```python
from build123d import *

# Parameters (mm, degrees)
F0_R      = 16
F0_R_2    = 15
F1_DEPTH  = 5
F2_R      = 16
F3_DEPTH  = 2
F4_R      = 3
F5_R      = 16
F6_DEPTH  = 1
F7_R      = 3
F8_R      = 5
F9_DEPTH  = 7
F10_R     = 6.15
F10_R_2   = 5.75
F11_DEPTH = 5


with BuildPart() as f1:
    # F0 (on Top) → F1 (new body)
    with BuildSketch(Plane.XY):
        Circle(F0_R)
        Circle(F0_R_2, mode=Mode.SUBTRACT)
    extrude(amount=F1_DEPTH)

    # F2 (on face) → F3 (join)
    with BuildSketch(Plane.XY.offset(5)):
        Circle(F2_R)
    extrude(amount=F3_DEPTH)

    # F4
    f4_edges = [f1.edges().sort_by_distance(p)[0] for p in [
        (-16, 0, 7),
    ]]
    fillet(f4_edges, radius=F4_R)

    # F5 (on face) → F6 (join)
    with BuildSketch(Plane(origin=(0, 0, 0), x_dir=(1, 0, 0), z_dir=(0, 0, -1))):
        Circle(F5_R)
    extrude(amount=F6_DEPTH)

    # F7
    f7_edges = [f1.edges().sort_by_distance(p)[0] for p in [
        (-16, 0, -1),
    ]]
    fillet(f7_edges, radius=F7_R)

    # F8 (on face) → F9 (cut)
    with BuildSketch(Plane.XY.offset(7)):
        Circle(F8_R)
    extrude(amount=-F9_DEPTH, mode=Mode.SUBTRACT)

    # F10 (on face) → F11 (join)
    with BuildSketch(Plane.XY.offset(7)):
        Circle(F10_R)
        Circle(F10_R_2, mode=Mode.SUBTRACT)
    extrude(amount=F11_DEPTH)

    # F13 (on Front) → F14 (revolve)
    with BuildSketch(Plane.XZ):
        with BuildLine():
            Line((0, 19.5), (0, 20))
            ThreePointArc((0, 20), (-9.192388, 16.192388), (-13, 7))
            Line((-13, 7), (-12.5, 7))
            ThreePointArc((-12.5, 7), (-8.838835, 15.838835), (0, 19.5))
        make_face()
    revolve(axis=Axis((0, 0, 13.5), (0, 0, 1)))


solid = f1.part
```
Work out the finished part from the listing and answer in its coordinate system (mm). Round coordinates to 2 decimals unless told otherwise and drop trailing zeros.
1) Consider probe 1 along Y at (x, z) = (0.5, 3); probe 2 along Z at (x, y) = (2, 8); probe 3 along Y at (x, z) = (0, 9.9). Determine where each line is inside the solid, lowest interval first.
2) Determine the mould class of faces 1 (the face through (0, 0, -1)), 2 (the face through (-3.47, 15.62, 3.01)), 3 (the face through (-1.08, -4.88, 6.01)) for opening direction Y: pulls with the +Y half, pulls with the -Y half, needs draft (parallel to the pull), parting line crosses it, or undercut.
3) A cutting plane is placed at A-A on z = 10.5. Give the number of separate pieces and of enclosed holes in the cut face, and give its area (3 significant figures).
4) Flat-ended cylindrical pins translate along their axes: P1, Ø1, axis at x = 6.5, y = -12, coming from the -Z side; P2, Ø8, axis at y = 0, z = 8, coming from the -X side; P3, Ø8, axis at x = -12, y = 10, coming from the +Z side; P4, Ø1.5, axis at y = -4, z = 12.5, coming from the +X side. Find the tip coordinate at first contact, or state that the pin passes through.
Entries:
1. probe 1: y = -15.99 to -14.99, 14.99 to 15.99
1. probe 2: z = -1 to 0, 5 to 7, 16.39 to 17.05
1. probe 3: y = -12.67 to -12.16, -6.15 to -5.75, 5.75 to 6.15, 12.16 to 12.67
2. face 1: needs draft
2. face 2: parting line crosses it
2. face 3: undercut
3. separate pieces: 2
3. enclosed holes: 2
3. area: 55.0 mm2
4. P1: stops at z = -1
4. P2: stops at x = -16
4. P3: stops at z = 12.83
4. P4: stops at x = 11.51
